Check sheet for the modelled part. Datum: model origin and axes. Units: mm. A direction names the side the tool comes from. Give positions to 0.01 mm unless a question says otherwise; leave off trailing zeros. Write each loop counter-clockwise with the first axis right and the second up, starting at its lowest first coordinate (ties: lowest second). Pieces come first, ordered by that corner, then holes. Notation, with made-up numbers: (63.5, 2) -> (95.5, 2) arc R18 ccw to (95.5, 24) -> close; hole circle Ø6 at (78.25, 66.25). An arc over 180 degrees is marked (long way). Write each question's results on one line, items separated by ' | '. Start each with the question number.
```python
from build123d import *

# Parameters (mm, degrees)
F1_DEPTH = 20


with BuildPart() as f1:
    # F0 (on Top) → F1 (new body)
    with BuildSketch(Plane.XY):
        with BuildLine():
            ThreePointArc((-44.90712, 13.333333), (-22.863558, 18.683447), (-10, 0))
            ThreePointArc((-10, 0), (-22.132295, -18.387475), (-43.809922, -14.466722))
            Line((-43.809922, -14.466722), (-30, -30))
            Line((-30, -30), (-17.320508, -30))
            ThreePointArc((-17.320508, -30), (0, -20), (17.320508, -30))
            Line((17.320508, -30), (30, -30))
            Line((30, -30), (30, 30))
            Line((30, 30), (20, 30))
            Line((20, 30), (0, 0))
            Line((0, 0), (-20, 30))
            Line((-20, 30), (-30, 30))
            Line((-30, 30), (-44.90712, 13.333333))
        make_face()
        with BuildLine():
            ThreePointArc((-43.809922, -14.466722), (-22.132295, -18.387475), (-10, 0))
            ThreePointArc((-10, 0), (-22.863558, 18.683447), (-44.90712, 13.333333))
            ThreePointArc((-44.90712, 13.333333), (-49.984441, -0.788735), (-43.809922, -14.466722))
        make_face()
    extrude(amount=F1_DEPTH)


solid = f1.part
```
Item 1: Section check A-A on y = 10. Record the boundary of the cut face in (x, z).
Item 2: Set-up check for faces 1 (the flat face through (10, 15, 10)), 2 (the flat face through (-25, 30, 10)): record each of +Z, -Z, +X, -X, +Y, -Y from which the full face is reachable in a straight line by a thin tool's end or side.
Item 3: Thickness scan on probe 1 along X at (y, z) = (12.5, 5.5); probe 2 along X at (y, z) = (18.5, 18.75); probe 3 along Y at (x, z) = (-5, 18.75). Record the ranges inside material, lowest first. Write a range as from..to.
Item 4: Section check B-B on z = 2.5. Record the boundary of the cut face in (x, y), then the cut area to 3 significant figures.
Item 5: Section check D-D on x = -35. Record the boundary of the cut face in (y, z), then the cut area to 3 significant figures.
Item 6: Section check C-C on y = -25. Record the boundary of the cut face in (x, z), then the cut area to 3 significant figures.
Item 7: Depth check by flat-ended pin: pin 1 Ø5 at (x, z) = (11, 11.5) entering from -Y; pin 2 Ø2 at (y, z) = (10, 10.5) entering from -X; pin 3 Ø5 at (y, z) = (8, 12.5) entering from -X. Enter the tip coordinate at first touch or a pass-through.
Item 8: Mould release check, pull along X, two halves, no side actions. Record for faces 3 (the flat face through (25, 30, 10)), 4 (the flat face through (-37.002, -22.125, 9.86)), 5 (the cylindrical face through (0, -20, 10)), 6 (the flat face through (30, 0, 10)): pulls with the +X half, pulls with the -X half, needs draft (parallel to the pull), parting line crosses it, or undercut.
Check sheet entries:
1) outline: (-47.32, 0) -> (-6.67, 0) -> (-6.67, 20) -> (-47.32, 20) -> close; (6.67, 0) -> (30, 0) -> (30, 20) -> (6.67, 20) -> close
2) face 1: +Z, -Z, +Y | face 2: +Z, -Z, +X, -X, +Y
3) probe 1: x = -45.61..-8.33, 8.33..30 | probe 2: x = -40.29..-12.33, 12.33..30 | probe 3: y = -20.64..7.5
4) outline: (-44.91, 13.33) arc R20 ccw to (-43.81, -14.47) -> (-30, -30) -> (-17.32, -30) arc R20 cw to (17.32, -30) -> (30, -30) -> (30, 30) -> (20, 30) -> (0, 0) -> (-20, 30) -> (-30, 30) -> close | area: 3,490 mm^2
5) outline: (-24.38, 0) -> (24.41, 0) -> (24.41, 20) -> (-24.38, 20) -> close | area: 976 mm^2
6) outline: (-34.45, 0) -> (-13.23, 0) -> (-13.23, 20) -> (-34.45, 20) -> close; (13.23, 0) -> (30, 0) -> (30, 20) -> (13.23, 20) -> close | area: 760 mm^2
7) pin 1: stops at y = -25.24 | pin 2: stops at x = -47.86 | pin 3: stops at x = -49.23
8) face 3: needs draft | face 4: pulls with the -X half | face 5: undercut | face 6: pulls with the +X half
